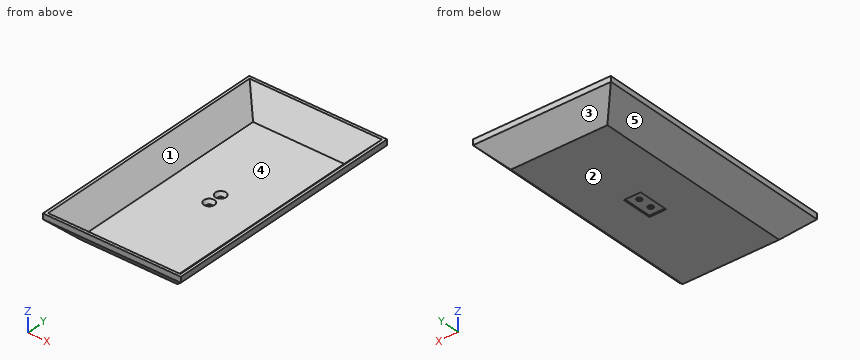
```python
from build123d import *

# Parameters (mm, degrees)
SKETCH_1_W               = 100
SKETCH_1_H               = 180
EXTRUDE_1_DEPTH          = 4
SKETCH_4_W               = 100
SKETCH_4_H               = 180
SKETCH_4_W_2             = 96
SKETCH_4_H_2             = 176
EXTRUDE_3_DEPTH          = 15
CHAMFER_1_SIZE           = 15
CUT_EXTRUDE_3_DEPTH      = 10
CUT_EXTRUDE_3_DEPTH_BACK = 105.694794522
SKETCH_6_R               = 1.9
CHAMFER_2_SIZE           = 2
CHAMFER_2_SIZE2          = 2.4
SKETCH_10_W              = 12.2
SKETCH_10_H              = 22.3
CUT_EXTRUDE_4_DEPTH      = 1


with BuildPart() as part:
    # 스케치1 → 보스-돌출1 (new body)
    with BuildSketch(Plane.XY):
        Rectangle(SKETCH_1_W, SKETCH_1_H)
    extrude(amount=EXTRUDE_1_DEPTH)

    # 스케치4 → 보스-돌출3 (add)
    with BuildSketch(Plane.XY.offset(4)):
        Rectangle(SKETCH_4_W, SKETCH_4_H)
        Rectangle(SKETCH_4_W_2, SKETCH_4_H_2, mode=Mode.SUBTRACT)
    extrude(amount=EXTRUDE_3_DEPTH)

    # 모따기1
    chamfer_1_edges = [part.edges().sort_by_distance(p)[0] for p in [
        (-48, 0, 4),
        (0, -88, 4),
        (50, 0, 0),
        (0, 90, 0),
        (-50, 0, 0),
        (0, -90, 0),
        (48, 0, 4),
        (0, 88, 4),
    ]]
    chamfer(chamfer_1_edges, length=CHAMFER_1_SIZE - 0.0001)  # a hair under: the kernel refuses the full size

    # 스케치6 → 컷-돌출3 (cut, two sides: drawn at the far end of the back side and taken through both)
    with BuildSketch(Plane.XY.offset(-CUT_EXTRUDE_3_DEPTH_BACK)):
        with Locations((0, 5)):
            Circle(SKETCH_6_R)
        with Locations((0, -5)):
            Circle(SKETCH_6_R)
    extrude(amount=CUT_EXTRUDE_3_DEPTH + CUT_EXTRUDE_3_DEPTH_BACK, mode=Mode.SUBTRACT)

    # 모따기2
    chamfer_2_edges = [part.edges().sort_by_distance(p)[0] for p in [
        (-1.9, 5, 4),
        (-1.9, -5, 4),
    ]]
    chamfer_2_side = [part.faces().sort_by_distance(p)[0] for p in [
        (0, 0, 4),
    ]]
    chamfer(chamfer_2_edges, length=CHAMFER_2_SIZE, length2=CHAMFER_2_SIZE2, reference=chamfer_2_side[0])

    # 스케치10 → 컷-돌출4 (cut)
    with BuildSketch(Plane(origin=(0, 0, 0), x_dir=(-1, 0, 0), z_dir=(0, 0, -1))):
        Rectangle(SKETCH_10_W, SKETCH_10_H)
    extrude(amount=-CUT_EXTRUDE_4_DEPTH, mode=Mode.SUBTRACT)


solid = part.part
```
Here's how the part is built. I have some questions about the finished solid (model axes, mm). Face numbers are marked on the shaded views. A direction names the side the tool comes from. Give positions to 0.01 mm unless a question says otherwise; leave off trailing zeros. Loops run counter-clockwise (first coordinate to the right, second up) from the corner with the lowest first, then second, coordinate; pieces in that order, holes last. Notation, with made-up numbers: (-26, 21.25) -> (-16, 21.25) arc R13 ccw to (-16, 44.25) -> close; hole circle Ø5 at (-23.75, 77). An arc over 180 degrees is marked (long way). Use one line per item in the form item = value. Start each with the question number.
1) For P1, Ø4, axis at y = 32.5, z = 3, coming from the +X side; P2, Ø1.1, axis at x = 0.5, z = 0.5, coming from the +Y side; P3, Ø6, axis at x = -7.5, z = 7, coming from the +Y side, each with a flat end and sliding along its axis, tell me the tip position at first contact or that it passes through.
2) Please list where these lines run through material, in increasing order: line 1 along Y through (x, z) = (0, 1.3); line 2 along Y through (x, z) = (0, 1.35); line 3 along Z through (x, y) = (14, 17.5).
3) Thinking about a two-plate mould opening in X: for the marked faces 3, 4 and 5, which applies, +X half, -X half, draft (parallel to the pull), parting line (faces both ways), or undercut?
4) Which directions (+Z, -Z, +X, -X, +Y, -Y) give clear straight access to the entire face, cutting with the end or side of a thin tool? Please do the marked faces 1 and 2.
5) Imagine slicing it at B-B (x = 0). Count the separate pieces of the cut face and the enclosed holes in it, then the cut area to 3 significant figures.
6) Imagine slicing it at C-C (z = 10.5). Please give me the cut outline in (x, y), then the cut area to 3 significant figures.
Check values:
q1.P1 = 40
q1.P2 = 76.05
q1.P3 = 85
q2.line_1 = -76.3 to -6.9, -3.1 to 3.1, 6.9 to 76.3
q2.line_2 = -76.35 to -6.9, -3.1 to 3.1, 6.9 to 76.35
q2.line_3 = 0 to 4
q3.face_3 = draft
q3.face_4 = undercut
q3.face_5 = -X half
q4.face_1 = +Z
q4.face_2 = -Z, +X, -X, +Y, -Y
q5.separate_pieces = 3
q5.enclosed_holes = 0
q5.area = 725 mm^2
q6.outline = (-45.5, -85.5) -> (45.5, -85.5) -> (45.5, 85.5) -> (-45.5, 85.5) -> close; hole (-39.5, -79.5) -> (39.5, -79.5) -> (39.5, 79.5) -> (-39.5, 79.5) -> close
q6.area = 3,000 mm^2
